```python
from build123d import *

# Parameters (mm, degrees)
SKICA1_R                 = 5.25
P_IDAT_VYSUNUT_M1_DEPTH  = 5
ZAOBLIT1_R               = 4
P_IDAT_VYSUNUT_M3_DEPTH  = 5
SKICA5_R                 = 4.25
SKICA5_R_2               = 1.75
P_IDAT_VYSUNUT_M4_DEPTH  = 1
SKICA8_R                 = 1.05
ODEBRAT_VYSUNUT_M3_DEPTH = 6
ODEBRAT_VYSUNUT_M4_DEPTH = 7
SKICA2_R                 = 1.75
ODEBRAT_VYSUNUT_M5_DEPTH = 10
SKICA10_R                = 3.5
ODEBRAT_VYSUNUT_M6_DEPTH = 3
ODEBRAT_START            = 50
SKICA11_R                = 0.75
ODEBRAT_VYSUNUT_M7_DEPTH = 10
P_IDAT_VYSUNUT_M5_DEPTH  = 10
P_IDAT_VYSUNUT_M6_DEPTH  = 8
ZAOBLIT2_R               = 2
ODEBRAT_VYSUNUT_M8_DEPTH = 7


with BuildPart() as part:
    # Skica1 → Přidat vysunutím1 (new body, symmetric)
    with BuildSketch(Plane.XY):
        with BuildLine():
            Line((0, 0), (0, 16))
            Line((0, 16), (24, 16))
            Line((24, 16), (24, 0))
            Line((24, 0), (29, 0))
            Line((29, 0), (97.312746067, 39.440382331))
            ThreePointArc((97.312746067, 39.440382331), (105.473420704, 36.802978572), (112.433277726, 41.81425579))
            Line((112.433277726, 41.81425579), (195.687578405, 27.134276321))
            ThreePointArc((195.687578405, 27.134276321), (209.374429572, 27.607666525), (196.674905514, 32.733686604))
            Line((196.674905514, 32.733686604), (113.420604835, 47.413666074))
            ThreePointArc((113.420604835, 47.413666074), (102.174688824, 55.511016714), (94.812746067, 43.77050935))
            Line((94.812746067, 43.77050935), (29, 5.773502692))
            Line((29, 5.773502692), (29, 21))
            Line((29, 21), (-5, 21))
            Line((-5, 21), (-5, 0))
            Line((-5, 0), (0, 0))
        make_face()
        with Locations((104, 46.188021535)):
            Circle(SKICA1_R, mode=Mode.SUBTRACT)
    extrude(amount=P_IDAT_VYSUNUT_M1_DEPTH, both=True)

    # Zaoblit1
    zaoblit1_edges = [part.edges().sort_by_distance(p)[0] for p in [
        (-5, 21, 0),
    ]]
    fillet(zaoblit1_edges, radius=ZAOBLIT1_R)

    # Skica4 → Přidat vysunutím3 (add, symmetric)
    with BuildSketch(Plane.XY):
        Polygon((29, 21), (66.969109888, 27.694978507), (59.37284323, 23.309271907), (29, 17.953720164), align=None)
    extrude(amount=P_IDAT_VYSUNUT_M3_DEPTH, both=True)

    # Skica5 → Přidat vysunutím4 (add)
    with BuildSketch(Plane.XY.offset(5)):
        with Locations((202.480775301, 28.823203768)):
            Circle(SKICA5_R)
        with Locations((202.480775301, 28.823203768)):
            Circle(SKICA5_R_2, mode=Mode.SUBTRACT)
    extrude(amount=P_IDAT_VYSUNUT_M4_DEPTH)

    # Skica8 → Odebrat vysunutím3 (cut)
    with BuildSketch(Plane.XZ):
        with Locations((-1.5, 0)):
            Circle(SKICA8_R)
        with Locations((25.5, 0)):
            Circle(SKICA8_R)
    extrude(amount=-ODEBRAT_VYSUNUT_M3_DEPTH, mode=Mode.SUBTRACT)

    # Skica9 → Odebrat vysunutím4 (cut)
    with BuildSketch(Plane.XY.offset(5)):
        Polygon((24, 16), (29, 16), (29, 13), (24, 8), align=None)
    extrude(amount=-ODEBRAT_VYSUNUT_M4_DEPTH, mode=Mode.SUBTRACT)

    # Skica2 → Odebrat vysunutím5 (cut)
    with BuildSketch(Plane.XY.offset(5)):
        with Locations((202.480775301, 28.823203768)):
            Circle(SKICA2_R)
    extrude(amount=-ODEBRAT_VYSUNUT_M5_DEPTH, mode=Mode.SUBTRACT)

    # Skica10 → Odebrat vysunutím6 (cut)
    with BuildSketch(Plane(origin=(0, 0, -5), x_dir=(-1, 0, 0), z_dir=(0, 0, -1))):
        with Locations((-202.480775301, 28.823203768)):
            Circle(SKICA10_R)
    extrude(amount=-ODEBRAT_VYSUNUT_M6_DEPTH, mode=Mode.SUBTRACT)


with BuildPart() as body_2:
    # Zrcadlit1: mirrored copy
    add(part.part.mirror(Plane(origin=(93.65445241, 28.310869093, -5), x_dir=(1, 0, 0), z_dir=(0, 0, -1))))

    # Skica11 → Odebrat vysunutím7 (cut)
    with BuildSketch(Plane(origin=(0, 0, 0), x_dir=(1, 0, 0), z_dir=(0, 1, 0)).offset(ODEBRAT_START)):
        with Locations((103.960302418, 10)):
            Circle(SKICA11_R)
    extrude(amount=ODEBRAT_VYSUNUT_M7_DEPTH, mode=Mode.SUBTRACT)

    # Skica12 → Přidat vysunutím5 (add)
    with BuildSketch(Plane(origin=(0, 0, -15), x_dir=(-1, 0, 0), z_dir=(0, 0, -1))):
        with BuildLine():
            Line((-209.480775301, 28.823203768), (-209.480775301, 16.823203768))
            Line((-209.480775301, 16.823203768), (-195.687578405, 16.823203768))
            Line((-195.687578405, 16.823203768), (-195.687578405, 27.134276321))
            ThreePointArc((-195.687578405, 27.134276321), (-203.331546047, 21.875096894), (-209.480775301, 28.823203768))
        make_face()
    extrude(amount=-P_IDAT_VYSUNUT_M5_DEPTH)

    # Skica13 → Přidat vysunutím6 (add)
    with BuildSketch(Plane(origin=(0, 0, -15), x_dir=(-1, 0, 0), z_dir=(0, 0, -1))):
        Polygon((-204.334176853, 20.823203768), (-200.834176853, 20.823203768), (-198.334176853, 16.823203768), (-206.834176853, 16.823203768), align=None)
    extrude(amount=P_IDAT_VYSUNUT_M6_DEPTH)

    # Zaoblit2
    zaoblit2_edges = [body_2.edges().sort_by_distance(p)[0] for p in [
        (195.687578405, 16.823203768, -10),
        (209.480775301, 16.823203768, -10),
    ]]
    fillet(zaoblit2_edges, radius=ZAOBLIT2_R)

    # Skica14 → Odebrat vysunutím8 (cut)
    with BuildSketch(Plane(origin=(0, 0, -15), x_dir=(-1, 0, 0), z_dir=(0, 0, -1))):
        Polygon((-59.37284323, 23.309271907), (-66.969109888, 27.694978507), (-61.786216453, 26.781094556), (-54.189949795, 22.395387956), align=None)
    extrude(amount=-ODEBRAT_VYSUNUT_M8_DEPTH, mode=Mode.SUBTRACT)


solid = body_2.part
```
The listing builds one solid part. Answer for the finished solid, in the listing's coordinates (mm). A direction names the side the tool comes from. Coordinates: 2 decimals unless noted, no trailing zeros. Write each loop counter-clockwise with the first axis right and the second up, starting at its lowest first coordinate (ties: lowest second). Pieces come first, ordered by that corner, then holes.
Q1. Which of the six approach directions +Z, -Z, +X, -X, +Y, -Y give full straight-line access (tool end or side, diameter ignored) to faces 1 (the flat face through (153.478, 34.577, -10.07)), 2 (the flat face through (18.7, 16.4, -15)), 3 (the flat face through (26, 13, -8))?
Returned:
face 1: +Z, -Z, -Y
face 2: -Z, -X, +Y, -Y
face 3: -Z
Q2. Section A-A, the plane z = -13 is taken. Write down the section's boundary in (x, y).
Returned:
outline: (-5, 0) - (0, 0) - (0, 16) - (29, 16) - (29, 17.95) - (54.19, 22.4) - (61.79, 26.78) - (29, 21) - (-1, 21) arc R4 ccw to (-5, 17) - close; (24, 0) - (29, 0) - (97.31, 39.44) arc R9.5 ccw to (112.43, 41.81) - (195.69, 27.13) - (195.69, 18.82) arc R2 ccw to (197.69, 16.82) - (207.48, 16.82) arc R2 ccw to (209.48, 18.82) - (209.48, 28.82) arc R7 ccw to (196.67, 32.73) - (113.42, 47.41) arc R9.5 ccw (long way) to (94.81, 43.77) - (29, 5.77) - (29, 13) - (24, 8) - close; hole circle Ø10.5 at (104, 46.19); hole circle Ø3.5 at (202.48, 28.82)
Q3. The mould has two halves that part along Y. Classify faces 4 (the flat face through (204, 30, -8)), 5 (the flat face through (203.4, 27, -16)), 6 (the flat face through (27, 0, -10)): released by +Y, released by -Y, zero draft, split by the parting line, or undercut.
Returned:
face 4: undercut
face 5: zero draft
face 6: released by -Y
Q4. Section C-C, the plane x = 163.5 is taken. Write down the section's boundary in (y, z).
Returned:
outline: (32.81, -15) - (38.58, -15) - (38.58, -5) - (32.81, -5) - close
Q5. Section B-B, the plane x = 13 is taken. Write down the section's boundary in (y, z).
Returned:
outline: (16, -15) - (21, -15) - (21, -5) - (16, -5) - close
Q6. Find the intervals of material crossed by line 1 along Z through (x, y) = (25.5, 4.4); line 2 along X through (y, z) = (4.4, -10); line 3 along X through (y, z) = (48.5, -11), in increasing order.
Returned:
line 1: z = -15 to -11.05, -8.95 to -5
line 2: x = -5 to -2.55, -0.45 to 0, 24 to 24.45, 26.55 to 36.62
line 3: x = 94.79 to 99.29, 108.71 to 113.21
Q7. Given P1, Ø4, axis at x = 202.5, z = -19.5, coming from the +Y side; P2, Ø8, axis at y = 14.5, z = -8.5, coming from the +X side; P3, Ø9.5, axis at x = 200.5, y = 29, coming from the -Z side; P4, Ø3, axis at x = 202.48, y = 28.82, coming from the +Z side, each flat-ended and moving along its own axis, determine where each tip first touches the part or whether it passes through.
Returned:
P1: stops at y = 20.82
P2: stops at x = 209.45
P3: stops at z = -16
P4: passes through
